Here's how the part is built. I have some questions about the finished solid (model axes, mm). Face numbers are marked on the shaded views. Give positions to 0.01 mm unless a question says otherwise; leave off trailing zeros. Loops run counter-clockwise (first coordinate to the right, second up) from the corner with the lowest first, then second, coordinate; pieces in that order, holes last.
Q1. If we section it at C-C (y = -19): Please give me the cut outline in (x, z).
Q2. Will these pins go through, and if not, where does the flat tip stop? P1, Ø4, axis at x = -1.5, y = -27, coming from the +Z side; P2, Ø3, axis at y = -46.5, z = -0.5, coming from the +X side; P3, Ø3, axis at y = -8.5, z = -3, coming from the +X side.
Q3. If we section it at A-A (z = 0): Please give me the cut outline in (x, y).
Q4. If we section it at B-B (x = 0): Please give me the cut outline in (y, z), plus the area to 3 significant figures.
Q5. We'd pull the mould along Y, two halves only. Please class the marked faces 1, 2 and 3: +Y half, -Y half, draft (parallel to the pull), parting line (faces both ways), or undercut.
Q6. I need wall thicknesses on line 1 (Y direction, x = 3.75, z = -0.75); line 2 (X direction, y = -20.5, z = 0.25). Which ranges of each line are inside material? Lowest first, please.
from build123d import *

# Parameters (mm, degrees)
SKETCH1_R           = 2.5
BOSS_EXTRUDE1_DEPTH = 58
SKETCH2_R           = 4
BOSS_EXTRUDE2_DEPTH = 5
BOSS_EXTRUDE3_START = -63
SKETCH3_R           = 4
BOSS_EXTRUDE3_DEPTH = 5


with BuildPart() as part:
    # Sketch1 → Boss-Extrude1 (new body)
    with BuildSketch(Plane(origin=(0, 0, 0), x_dir=(1, 0, 0), z_dir=(0, 1, 0))):
        with Locations(Location((0, 0, 0), (0, 0, 270))):
            Circle(SKETCH1_R)
    extrude(amount=-BOSS_EXTRUDE1_DEPTH)

    # Sketch2 → Boss-Extrude2 (add)
    with BuildSketch(Plane(origin=(0, 0, 0), x_dir=(1, 0, 0), z_dir=(0, 1, 0))):
        with Locations(Location((0, 0, 0), (0, 0, 270))):
            Circle(SKETCH2_R)
    extrude(amount=BOSS_EXTRUDE2_DEPTH)

    # Sketch3 → Boss-Extrude3 (add)
    with BuildSketch(Plane(origin=(0, 0, 0), x_dir=(1, 0, 0), z_dir=(0, 1, 0)).offset(BOSS_EXTRUDE3_START)):
        with Locations(Location((0, 0, 0), (0, 0, 270))):
            Circle(SKETCH3_R)
    extrude(amount=BOSS_EXTRUDE3_DEPTH)


solid = part.part
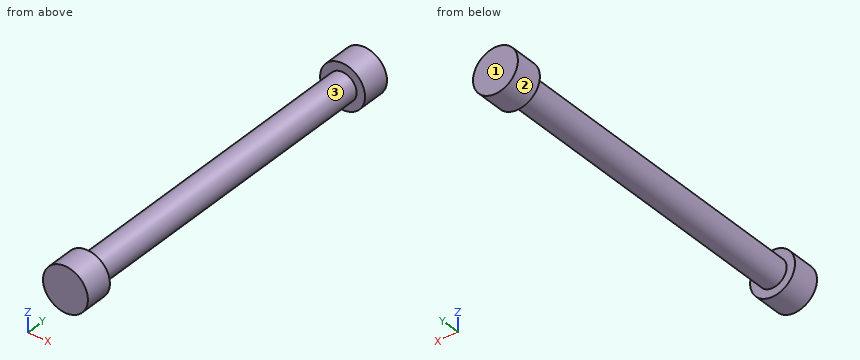
Check sheet entries:
1. outline: circle Ø5 at (0, 0)
2. P1: stops at z = 2.5
2. P2: stops at x = 2.5
2. P3: stops at x = 2
3. outline: (-4, -63) - (4, -63) - (4, -58) - (2.5, -58) - (2.5, 0) - (4, 0) - (4, 5) - (-4, 5) - (-4, 0) - (-2.5, 0) - (-2.5, -58) - (-4, -58) - close
4. outline: (-63, -4) - (-58, -4) - (-58, -2.5) - (0, -2.5) - (0, -4) - (5, -4) - (5, 4) - (0, 4) - (0, 2.5) - (-58, 2.5) - (-58, 4) - (-63, 4) - close
4. area: 370 mm2
5. face 1: +Y half
5. face 2: draft
5. face 3: undercut
6. line 1: y = -63 to -58, 0 to 5
6. line 2: x = -2.49 to 2.49
